Autodesk Inventor part; units mm, degrees
ref_plane "YZ Plane" through (0, 0, 0) normal (1, 0, 0) x (0, 1, 0)
ref_plane "XZ Plane" through (0, 0, 0) normal (0, 1, 0) x (-1, 0, 0)
ref_plane "XY Plane" through (0, 0, 0) normal (0, 0, 1) x (1, 0, 0)
sketch "Sketch2" plane through (0, 0, 0) normal (0, 1, 0) x (-1, 0, 0)
  line L0 (35, -35) -> (-35, -35)
  line L1 (-35, -35) -> (-35, 35)
  line L2 (-35, 35) -> (35, 35)
  line L3 (35, 35) -> (35, -35)
  line L4 (35, -35) -> (-35, 35) construction
  line L5 (-35, -35) -> (35, 35) construction
  line L6 (25, 25) -> (-25, 25)
  line L7 (-25, 25) -> (-25, -25)
  line L8 (-25, -25) -> (25, -25)
  line L9 (25, -25) -> (25, 25)
  point P0 (0, 0)
  dimension "d0" = 70
  dimension "d1" = 10
  dimension "d27" = 70
extrude "Extrusion1" add sketch "Sketch2" along normal blind 5
chamfer "Chamfer1" distance 10 angle 45 8 edges at (-25, 2.5, 25) (25, 2.5, 25) (-25, 2.5, -25) (25, 2.5, -25) (-35, 2.5, 35) (35, 2.5, 35) (35, 2.5, -35) (-35, 2.5, -35)
sketch "Sketch3" plane through (0, 5, 0) normal (0, 1, 0) x (1, 0, 0)
  line L0 (-35, 25) -> (-35, -25) construction
  line L1 (25, 35) -> (-25, 35) construction
  circle A0 centre (-25, 25) radius 2.5
  point P0 (0, 0)
  dimension "d7" = 10
  dimension "d8" = 10
  dimension "d9" = 5
extrude "Extrusion2" cut sketch "Sketch3" against normal through all
pattern_circular "Circular Pattern1" count 4 over 360 about axis through (0, -10, 0) along (0, 1, 0) of "Extrusion2"
sketch "Sketch4" plane through (0, 0, 0) normal (0, 0, 1) x (1, 0, 0)
  line L0 (-35, 5) -> (-35, 0) construction
  line L1 (-35, 5) -> (-25, 5)
  line L2 (-25, 5) -> (-25, 15)
  line L3 (-25, 15) -> (-35, 15)
  line L4 (-35, 15) -> (-35, 5)
  point P0 (0, 0)
  dimension "d15" = 10
  dimension "d16" = 10
extrude "Extrusion3" add sketch "Sketch4" along normal mid plane 30
sketch "Sketch6" plane through (0, 0, 0) normal (0, 0, 1) x (1, 0, 0)
  circle A0 centre (-30, 10) radius 2.5
  line L0 (-25, 15) -> (-35, 15) construction
  line L1 (-35, 15) -> (-35, 5) construction
  line L2 (-27.5, 5) -> (-22.5, 5) construction
  line L3 (-35, 15) -> (-25, 15)
  line L4 (-25, 15) -> (-25, 5)
  line L5 (-25, 5) -> (-35, 5)
  line L6 (-35, 5) -> (-35, 15)
  point P0 (0, 0)
  point P1 (-30, 15)
  point P2 (-35, 10)
  dimension "d22" = 5
  dimension "d23" = 5
  dimension "d24" = 5
extrude "Extrusion4" cut sketch "Sketch6" along normal mid plane 20
sketch "Sketch7" plane through (35, 0, 25) normal (1, 0, 0) x (0, 0, -1)
  line L0 (50, 5) -> (50, 0) construction
  line L1 (16.3397, 5) -> (25, 10)
  line L2 (25, 10) -> (33.6603, 5)
  line L3 (33.6603, 5) -> (33.6603, -5)
  line L4 (33.6603, -5) -> (25, -10)
  line L5 (25, -10) -> (16.3397, -5)
  line L6 (16.3397, -5) -> (16.3397, 5)
  point P0 (25, 0)
  point P1 (25, 0)
  dimension "d28" = 10
extrude "Extrusion5" cut sketch "Sketch7" against normal blind 10
fillet "Fillet1" radius 5 4 edges at (-35, 15, 12.5) (-25, 15, 12.5) (-35, 15, -12.5) (-25, 15, -12.5)
chamfer "Chamfer2" distance 1 angle 45 4 edges at (-25, 5, 27.5) (-27.5, 5, -25) (25, 5, -27.5) (27.5, 5, 25)
properties part number "pokemon_ball_black_part1"
The model under review builds one solid part; all positions refer to its coordinate system, in mm. A direction names the side the tool comes from. Round coordinates to 2 decimals unless told otherwise and drop trailing zeros. Write each loop counter-clockwise with the first axis right and the second up, starting at its lowest first coordinate (ties: lowest second). Pieces come first, ordered by that corner, then holes. Notation, with made-up numbers: M 35.25,-22.5 L 39.25,-22.5 A16 cw 39.25,-7.5 Z; hole C -2,21.25 d11. An arc over 180 degrees is marked long. Use CSV: the item, a comma, the result in double quotes. Start each with the question number.
(1) For line 1 along Z through (x, y) = (10.5, 1.25); line 2 along Z through (x, y) = (-30, 14); line 3 along X through (y, z) = (3.5, 25.5), list the stretches that pass through material, from the lowest coordinate up.
(2) We need section C-C, the plane y = 2.5. State the section outline as (x, z) points.
(3) We need section D-D, the plane x = -5. State the section outline as (y, z) points.
(4) We need section A-A, the plane x = -18. State the section outline as (y, z) points.
(5) The part is to be moulded in two halves that separate along X. For faces 1 (the face through (25, 2, 12)), 2 (the face through (-34, 13, 12)), 3 (the face through (-27, 14, 12)), 4 (the face through (-26, 0, -2)), say which applies: +X half, -X half, draft (parallel to the pull), parting line (faces both ways), or undercut.
(6) We need section B-B, the plane z = 0. State the section outline as (x, y) points, then the cut area to 3 significant figures.
(7) Tool access review of faces 5 (the face through (-25, 4, 0)), 6 (the face through (-27, 14, -13)): name each direction out of +Z, -Z, +X, -X, +Y, -Y from which nothing blocks a thin tool from reaching the whole face with its end or side.
(8) Clearance check with flat-ended pins moving along their axes: P1, Ø13, axis at x = -7, z = -19, coming from the +Y side; P2, Ø5, axis at x = -27.5, y = 10.5, coming from the +Z side; P3, Ø4, axis at x = 30, y = 2.5, coming from the -Z side; P4, Ø3, axis at x = 25, z = 25, coming from the -Y side. State where each tip first meets the part, or that it passes through.
Findings:
1,line 1,"-35 to -25, 25 to 35"
1,line 2,"-15 to -10, 10 to 15"
1,line 3,"-34.5 to -27.45, -22.55 to 22.55, 27.45 to 34.5"
2,outline,"M -35,-25 L -25,-35 L 25,-35 L 35,-25 L 35,-8.66 L 25,-8.66 L 25,-15 L 15,-25 L -15,-25 L -25,-15 L -25,15 L -15,25 L 15,25 L 25,15 L 25,8.66 L 35,8.66 L 35,25 L 25,35 L -25,35 L -35,25 Z; hole C -25,-25 d5; hole C -25,25 d5; hole C 25,-25 d5; hole C 25,25 d5"
3,outline,"M 0,-35 L 5,-35 L 5,-25 L 0,-25 Z; M 0,25 L 5,25 L 5,35 L 0,35 Z"
4,outline,"M 0,-35 L 5,-35 L 5,-22 L 0,-22 Z; M 0,22 L 5,22 L 5,35 L 0,35 Z"
5,face 1,"undercut"
5,face 2,"-X half"
5,face 3,"+X half"
5,face 4,"draft"
6,outline,"M -35,0 L -25,0 L -25,5 L -35,5 Z; C -30,10 d5"
6,area,"69.6 mm^2"
7,face 5,"+Y, -Y"
7,face 6,"+Z, -Z, +X, +Y"
8,P1,"y = 5"
8,P2,"z = 15"
8,P3,"z = -32"
8,P4,"through"
